```python
from build123d import *

# Parameters (mm, degrees)
F1_DEPTH = 10


with BuildPart() as f1:
    # F0 (on Top) → F1 (new body)
    with BuildSketch(Plane.XY):
        with BuildLine():
            Line((70, 7.5), (-85, 7.5))
            Line((-85, 7.5), (-85, 2))
            ThreePointArc((-85, 2), (-83.585786, 1.414214), (-83, 0))
            ThreePointArc((-83, 0), (-83.585786, -1.414214), (-85, -2))
            Line((-85, -2), (-85, -7.5))
            Line((-85, -7.5), (70, -7.5))
            Line((70, -7.5), (77.5, 0))
            Line((77.5, 0), (70, 7.5))
        make_face()
        with BuildLine():
            Line((-85, 2), (-85, 7.5))
            ThreePointArc((-85, 7.5), (-92.5, 0), (-85, -7.5))
            Line((-85, -7.5), (-85, -2))
            ThreePointArc((-85, -2), (-87, 0), (-85, 2))
        make_face()
    extrude(amount=F1_DEPTH)


solid = f1.part
```
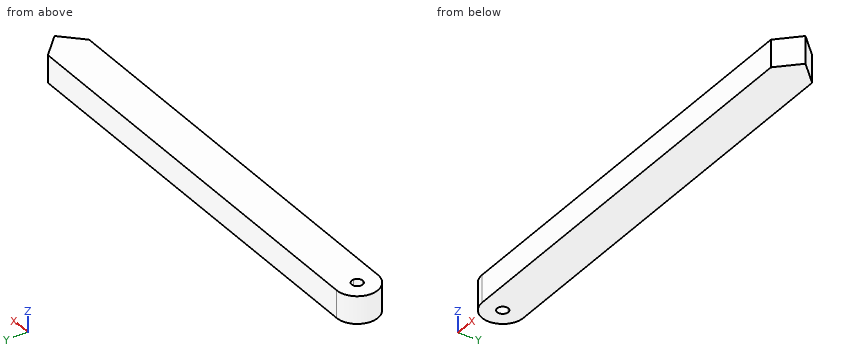
Geometry: final body of the model. Coordinates: model frame, mm. Round coordinates to 2 decimals unless told otherwise and drop trailing zeros. Order: outer loops, then holes, each group sorted by start corner. A loop starts at its lowest first (then second) coordinate and runs counter-clockwise, first axis right, second up. Notation, with made-up numbers: (58.5, 7.25) - (93.5, 7.25) arc R23 cw to (93.5, 43.25) - close; hole circle Ø9 at (77.5, -17). An arc over 180 degrees is marked (long way). Write item = value, one per line. Start each with the question number.
Q1. Ray query, line 1 (X direction, y = -0.75, z = 5.5); line 2 (X direction, y = -4.25, z = 2.75). Return the intervals inside material, ascending. Write a range as from..to.
Q2. Cut plane C-C on y = 4.75. Return the cut outline in (x, z), and give its area (3 significant figures).
Q3. Cut plane A-A on z = 4.25. Return the cut outline in (x, y).
Q4. Cut plane B-B on y = -5. Return the cut outline in (x, z), and give its area (3 significant figures).
Q5. Pin query (flat end, axial travel): pin 1 (5 mm diameter, centred on y = -3, z = 5.5, fed in from +X). Return the tip coordinate at first contact, or that it passes through.
Outcome:
q1.line_1 = -92.46..-86.85, -83.15..76.75
q1.line_2 = -91.18..73.25
q2.outline = (-90.8, 0) - (72.75, 0) - (72.75, 10) - (-90.8, 10) - close
q2.area = 1,640 mm^2
q3.outline = (-85, -7.5) - (70, -7.5) - (77.5, 0) - (70, 7.5) - (-85, 7.5) arc R7.5 ccw to start; hole (-85, -2) arc R2 ccw to (-83, 0) arc R2 ccw to (-85, 2) arc R2 ccw to start
q4.outline = (-90.59, 0) - (72.5, 0) - (72.5, 10) - (-90.59, 10) - close
q4.area = 1,630 mm^2
q5.pin_1 = 77
